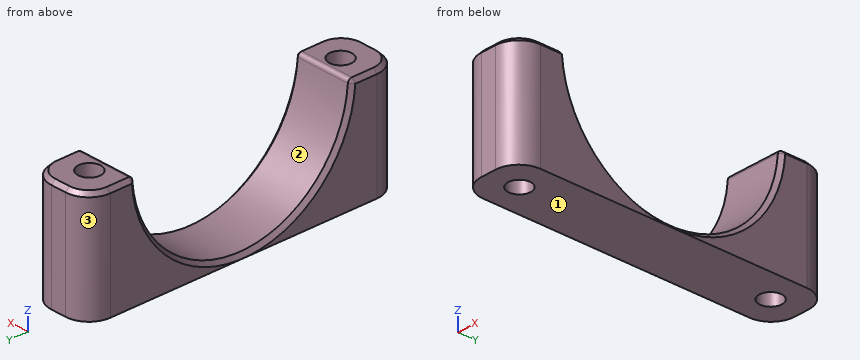
from build123d import *

# Parameters (mm, degrees)
SKETCH_1_R               = 1.45
EXTRUDE_1_DEPTH          = 14
CUT_EXTRUDE_1_DEPTH      = 26.896554891
CUT_EXTRUDE_1_DEPTH_BACK = 26.896554891
SKETCH_2_R               = 14
FILLET_1_R               = 0.5
CHAMFER_1_SIZE           = 0.5


with BuildPart() as part:
    # 草图1 → 凸台-拉伸1 (new body)
    with BuildSketch(Plane.XY):
        with BuildLine():
            Line((151.264880132, 20.264045876), (153.264880132, 20.264045876))
            ThreePointArc((153.264880132, 20.264045876), (155.386200475, 19.385366219), (156.264880132, 17.264045876))
            Line((156.264880132, 17.264045876), (156.264880132, -17.264045876))
            ThreePointArc((156.264880132, -17.264045876), (155.386200475, -19.385366219), (153.264880132, -20.264045876))
            Line((153.264880132, -20.264045876), (151.264880132, -20.264045876))
            ThreePointArc((151.264880132, -20.264045876), (149.143559788, -19.385366219), (148.264880132, -17.264045876))
            Line((148.264880132, -17.264045876), (148.264880132, 17.264045876))
            ThreePointArc((148.264880132, 17.264045876), (149.143559788, 19.385366219), (151.264880132, 20.264045876))
        make_face()
        with Locations((152.264880132, 16.264045876)):
            Circle(SKETCH_1_R, mode=Mode.SUBTRACT)
        with Locations((152.264880132, -16.264045876)):
            Circle(SKETCH_1_R, mode=Mode.SUBTRACT)
    extrude(amount=EXTRUDE_1_DEPTH)

    # 草图2 → 切除-拉伸1 (cut, two sides: drawn at the far end of the back side and taken through both)
    with BuildSketch(Plane.ZY.offset(-148.264880132).offset(-CUT_EXTRUDE_1_DEPTH_BACK)):
        with Locations((14.5, 0)):
            Circle(SKETCH_2_R)
    extrude(amount=CUT_EXTRUDE_1_DEPTH + CUT_EXTRUDE_1_DEPTH_BACK, mode=Mode.SUBTRACT)

    # 圆角1
    fillet_1_edges = [part.edges().sort_by_distance(p)[0] for p in [
        (152.264880132, 13.99106858, 14),
        (152.264880132, -13.99106858, 14),
    ]]
    fillet(fillet_1_edges, radius=FILLET_1_R)

    # 倒角1
    chamfer_1_edges = [part.edges().sort_by_distance(p)[0] for p in [
        (155.386200475, 19.385366219, 14),
        (152.264880132, 20.264045876, 14),
        (149.143559788, 19.385366219, 14),
        (148.264880132, 15.864761009, 14),
        (149.143559788, -19.385366219, 14),
        (152.264880132, -20.264045876, 14),
        (148.264880132, 0, 0.5),
        (156.264880132, 0, 0.5),
        (156.264880132, 15.864761009, 14),
        (156.264880132, 14.124332022, 13.865541639),
        (156.264880132, -14.124332022, 13.865541639),
        (148.264880132, -15.864761009, 14),
        (148.264880132, 14.124332022, 13.865541639),
        (148.264880132, -14.124332022, 13.865541639),
        (155.386200475, -19.385366219, 14),
        (156.264880132, -15.864761009, 14),
    ]]
    chamfer(chamfer_1_edges, length=CHAMFER_1_SIZE - 0.0001)  # a hair under: the kernel refuses the full size


solid = part.part
Model file for the job. Use its own axes, mm. Face numbers are marked on the shaded views. Coordinates: 2 decimals unless noted, no trailing zeros. Order: outer loops, then holes, each group sorted by start corner. A loop starts at its lowest first (then second) coordinate and runs counter-clockwise, first axis right, second up. Notation, with made-up numbers: M 70,-15.75 L 98,-15.75 A20 ccw 98,5.25 Z; hole C 10.5,-30 d2. An arc over 180 degrees is marked long. Return JSON: item names as keys, results as strings.
1. Saw through at B-B (z = 1.5). Give the number of separate pieces and of enclosed holes in the cut face, and give its area (3 significant figures).
Ans:
{"separate pieces": "2", "enclosed holes": "2", "area": "219 mm^2"}
2. Drill centre lines: probe 1 along Y at (x, z) = (153, 11.5); probe 2 along Y at (x, z) = (151.5, 9.5); probe 3 along Y at (x, z) = (150.25, 1.75). Where is each one in solid material? Low to high.
Ans:
{"probe 1": "-20.26 to -17.51, -15.01 to -13.67, 13.67 to 15.01, 17.51 to 20.26", "probe 2": "-20.26 to -17.5, -15.03 to -13.08, 13.08 to 15.03, 17.5 to 20.26", "probe 3": "-20.09 to -5.78, 5.78 to 20.09"}
3. Pull direction Y, two halves, no side cores. Call the marked faces 1, 2 and 3: +Y half, -Y half, draft (parallel to the pull), parting line (faces both ways), or undercut.
Ans:
{"face 1": "draft", "face 2": "undercut", "face 3": "+Y half"}
4. Saw through at A-A (x = 152.75). Give the cut face in (y, z), and give its area (3 significant figures).
Ans:
{"outline": "M -20.26,0 L -17.63,0 L -17.63,14 L -19.76,14 L -20.26,13.5 Z; M -14.9,0 L 14.9,0 L 14.9,14 L 14.47,14 A0.5 ccw 13.97,13.53 A14 cw -13.97,13.53 A0.5 ccw -14.47,14 L -14.9,14 Z; M 17.63,0 L 20.26,0 L 20.26,13.5 L 19.76,14 L 17.63,14 Z", "area": "197 mm^2"}
5. Flat gauge pin, fed straight in: pin 1 (2.5 mm diameter, centred on x = 152.26, y = -16.26, fed in from -Z). Where does the tip first touch, or does it go through?
Ans:
{"pin 1": "through"}
